Verification items for the finished model (mm, model axes). Give positions to 0.01 mm unless a question says otherwise; leave off trailing zeros. Write each loop counter-clockwise with the first axis right and the second up, starting at its lowest first coordinate (ties: lowest second). Pieces come first, ordered by that corner, then holes. Notation, with made-up numbers: (38, 40.25) -> (76, 40.25) arc R17 ccw to (76, 55.25) -> close; hole circle Ø9 at (9, 59). An arc over 180 degrees is marked (long way). Use CSV: the item, a comma, the result in double quotes. Start each with the question number.
```python
from build123d import *

# Parameters (mm, degrees)
SKETCH1_W           = 8.38
SKETCH1_H           = 21.2
BOSS_EXTRUDE1_DEPTH = 2.36
SKETCH2_W           = 0.41
SKETCH2_H           = 0.41
BOSS_EXTRUDE2_DEPTH = 3.05
SKETCH3_W           = 0.65
SKETCH3_H           = 0.65
CUT_EXTRUDE1_DEPTH  = 3.05


with BuildPart() as part:
    # Sketch1 → Boss-Extrude1 (new body)
    with BuildSketch(Plane(origin=(0, 0, 0), x_dir=(1, 0, 0), z_dir=(0, 1, 0))):
        with Locations((4.19, 10.6)):
            Rectangle(SKETCH1_W, SKETCH1_H)
    extrude(amount=BOSS_EXTRUDE1_DEPTH)

    # Sketch2 → Boss-Extrude2 (add)
    with BuildSketch(Plane(origin=(8.38, 0, 0), x_dir=(0, 0, -1), z_dir=(1, 0, 0))):
        with Locations((1.58, 1.18)):
            Rectangle(SKETCH2_W, SKETCH2_H)
        with Locations((4.157142857, 1.18)):
            Rectangle(SKETCH2_W, SKETCH2_H)
        with Locations((6.734285714, 1.18)):
            Rectangle(SKETCH2_W, SKETCH2_H)
        with Locations((9.311428571, 1.18)):
            Rectangle(SKETCH2_W, SKETCH2_H)
        with Locations((11.888571429, 1.18)):
            Rectangle(SKETCH2_W, SKETCH2_H)
        with Locations((14.465714286, 1.18)):
            Rectangle(SKETCH2_W, SKETCH2_H)
        with Locations((17.042857143, 1.18)):
            Rectangle(SKETCH2_W, SKETCH2_H)
        with Locations((19.62, 1.18)):
            Rectangle(SKETCH2_W, SKETCH2_H)
    extrude(amount=BOSS_EXTRUDE2_DEPTH)

    # Sketch3 → Cut-Extrude1 (cut)
    with BuildSketch(Plane.ZY):
        with Locations((-19.475, 1.18)):
            Rectangle(SKETCH3_W, SKETCH3_H)
        with Locations((-16.939285714, 1.18)):
            Rectangle(SKETCH3_W, SKETCH3_H)
        with Locations((-14.403571429, 1.18)):
            Rectangle(SKETCH3_W, SKETCH3_H)
        with Locations((-11.867857143, 1.18)):
            Rectangle(SKETCH3_W, SKETCH3_H)
        with Locations((-9.332142857, 1.18)):
            Rectangle(SKETCH3_W, SKETCH3_H)
        with Locations((-6.796428571, 1.18)):
            Rectangle(SKETCH3_W, SKETCH3_H)
        with Locations((-4.260714286, 1.18)):
            Rectangle(SKETCH3_W, SKETCH3_H)
        with Locations((-1.725, 1.18)):
            Rectangle(SKETCH3_W, SKETCH3_H)
    extrude(amount=-CUT_EXTRUDE1_DEPTH, mode=Mode.SUBTRACT)


solid = part.part
```
(1) Section check A-A on x = 9.25. Give the number of separate pieces and of enclosed holes in the cut face, then the cut area to 3 significant figures.
(2) Thickness scan on line 1 (X direction, y = 0.65, z = -19.5); line 2 (Y direction, x = 8.75, z = -19.75) (3 decimals); line 3 (X direction, y = 0.9, z = -4). Record the ranges inside material, lowest first. Write a range as from..to.
(3) Section check C-C on y = 1.7. Record the cut outline in (x, z).
(4) Section check D-D on z = -6.25. Record the cut outline in (x, y).
(5) Go/stop test with flat-tipped pins: pin 1 (0.5 mm diameter, centred on x = 10.5, y = 1, fed in from +Z) (3 decimals); pin 2 (0.7 mm diameter, centred on y = 1, z = -2, fed in from -X); pin 3 (0.5 mm diameter, centred on x = 10, y = 1, fed in from -Z) (3 decimals); pin 4 (1 mm diameter, centred on x = 9, y = 2, fed in from -Z). Record where each tip stops, or that it passes through.
Data:
1,separate pieces,"8"
1,enclosed holes,"0"
1,area,"1.34 mm2"
2,line 1,"x = 0..8.38"
2,line 2,"y = 0.975..1.385"
2,line 3,"x = 3.05..8.38"
3,outline,"(0, -21.2) -> (8.38, -21.2) -> (8.38, 0) -> (0, 0) -> close"
4,outline,"(0, 0) -> (8.38, 0) -> (8.38, 2.36) -> (0, 2.36) -> close"
5,pin 1,"stops at z = -1.375"
5,pin 2,"stops at x = 0"
5,pin 3,"stops at z = -19.825"
5,pin 4,"passes through"
